For this review, take the finished solid that the model builds, in its own axes (mm). Face numbers are marked on the shaded views. A direction names the side the tool comes from. Give positions to 0.01 mm unless a question says otherwise; leave off trailing zeros. Write each loop counter-clockwise with the first axis right and the second up, starting at its lowest first coordinate (ties: lowest second). Pieces come first, ordered by that corner, then holes. Notation, with made-up numbers: (39.25, 23.25) -> (98.25, 23.25) arc R30 ccw to (98.25, 59.25) -> close; hole circle Ø4 at (-18.75, 42). An arc over 180 degrees is marked (long way). Return JSON: item names as keys, results as strings.
from build123d import *

# Parameters (mm, degrees)
F1_DEPTH = 57.15
F2_R     = 12.7
F3_DEPTH = 44.45
F4_R     = 5.08
F5_DEPTH = 25.4


with BuildPart() as f1:
    # F0 (on Front) → F1 (new body)
    with BuildSketch(Plane.XZ):
        with BuildLine():
            Line((0, 12.7), (0, 0))
            Line((0, 0), (63.5, 0))
            Line((63.5, 0), (63.5, 12.7))
            Line((63.5, 12.7), (44.45, 12.7))
            Line((44.45, 12.7), (44.45, 21.59))
            Line((44.45, 21.59), (95.25, 21.59))
            Line((95.25, 21.59), (95.25, 34.29))
            Line((95.25, 34.29), (79.375, 34.29))
            Line((79.375, 34.29), (52.843426, 73.840173))
            ThreePointArc((52.843426, 73.840173), (43.702941, 82.101765), (31.75, 85.09))
            ThreePointArc((31.75, 85.09), (19.797059, 82.101765), (10.656574, 73.840173))
            Line((10.656574, 73.840173), (-15.875, 34.29))
            Line((-15.875, 34.29), (-31.75, 34.29))
            Line((-31.75, 34.29), (-31.75, 21.59))
            Line((-31.75, 21.59), (19.05, 21.59))
            Line((19.05, 21.59), (19.05, 12.7))
            Line((19.05, 12.7), (0, 12.7))
        make_face()
        with BuildLine():
            Line((-31.75, 85.09), (-31.75, 34.29))
            Line((-31.75, 34.29), (-15.875, 34.29))
            Line((-15.875, 34.29), (10.656574, 73.840173))
            ThreePointArc((10.656574, 73.840173), (19.797059, 82.101765), (31.75, 85.09))
            Line((31.75, 85.09), (-31.75, 85.09))
        make_face()
        with BuildLine():
            Line((79.375, 34.29), (95.25, 34.29))
            Line((95.25, 34.29), (95.25, 85.09))
            Line((95.25, 85.09), (31.75, 85.09))
            ThreePointArc((31.75, 85.09), (43.702941, 82.101765), (52.843426, 73.840173))
            Line((52.843426, 73.840173), (79.375, 34.29))
        make_face()
    extrude(amount=F1_DEPTH)

    # F2 (on face) → F3 (cut)
    with BuildSketch(Plane.XZ.offset(57.15)):
        with BuildLine():
            Line((-31.75, 85.09), (-31.75, 34.29))
            Line((-31.75, 34.29), (-16.115654, 34.29))
            Line((-16.115654, 34.29), (10.664181, 74.163921))
            ThreePointArc((10.664181, 74.163921), (18.082063, 81.411466), (27.778468, 85.09))
            Line((27.778468, 85.09), (-31.75, 85.09))
        make_face()
        with BuildLine():
            Line((95.25, 85.09), (35.721532, 85.09))
            ThreePointArc((35.721532, 85.09), (45.417937, 81.411466), (52.835819, 74.163921))
            Line((52.835819, 74.163921), (79.615654, 34.29))
            Line((79.615654, 34.29), (95.25, 34.29))
            Line((95.25, 34.29), (95.25, 85.09))
        make_face()
        with BuildLine():
            ThreePointArc((35.721532, 85.09), (31.75, 85.402415), (27.778468, 85.09))
            Line((27.778468, 85.09), (35.721532, 85.09))
        make_face()
        with Locations((31.75, 60.002415)):
            Circle(F2_R)
    extrude(amount=-F3_DEPTH, mode=Mode.SUBTRACT)

    # F4 (on face) → F5 (cut)
    with BuildSketch(Plane.XY.offset(85.09)):
        with Locations((31.75, -34.925)):
            Circle(F4_R)
    extrude(amount=-F5_DEPTH, mode=Mode.SUBTRACT)


solid = f1.part
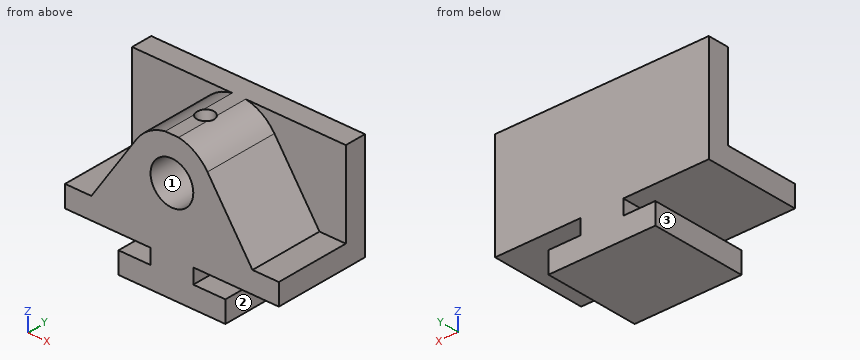
1. To check wall thickness, follow probe 1 along Z at (x, y) = (52, -8.5); probe 2 along Z at (x, y) = (31.75, -45); probe 3 along Y at (x, z) = (31.75, 75.25) (3 decimals). State the ranges of each line that lie inside material, in increasing order.
Results found:
{"probe 1": "z = 0 to 12.7, 21.59 to 85.09", "probe 2": "z = 0 to 47.3, 72.7 to 85.09", "probe 3": "y = -57.15 to -40.005, -29.845 to 0"}
2. Add section B-B, the plane y = -25. State the section outline as (x, z) points, plus the area to 3 significant figures.
Results found:
{"outline": "(-31.75, 21.59) -> (19.05, 21.59) -> (19.05, 12.7) -> (0, 12.7) -> (0, 0) -> (63.5, 0) -> (63.5, 12.7) -> (44.45, 12.7) -> (44.45, 21.59) -> (95.25, 21.59) -> (95.25, 34.29) -> (79.62, 34.29) -> (52.84, 74.16) arc R25.4 ccw to (35.72, 85.09) -> (27.78, 85.09) arc R25.4 ccw to (10.66, 74.16) -> (-16.12, 34.29) -> (-31.75, 34.29) -> close; hole circle Ø25.4 at (31.75, 60)", "area": "5,220 mm²"}
3. Add section C-C, the plane z = 11. State the section outline as (x, y) points.
Results found:
{"outline": "(0, -57.15) -> (63.5, -57.15) -> (63.5, 0) -> (0, 0) -> close"}
4. For the marked faces 1, 2 and 3, list the 3-axis set-ups (+Z, -Z, +X, -X, +Y, -Y) from which the entire face can be reached by the end or side of a thin tool; tool diameter is ignored.
Results found:
{"face 1": "-Y", "face 2": "-Z, +X, +Y, -Y", "face 3": "-Z, -X, +Y, -Y"}
5. Add section A-A, the plane x = 31.75. State the section outline as (y, z) points (3 decimals).
Results found:
{"outline": "(-57.15, 0) -> (0, 0) -> (0, 85.09) -> (-29.845, 85.09) -> (-29.845, 72.702) -> (-12.7, 72.702) -> (-12.7, 47.302) -> (-57.15, 47.302) -> close; (-57.15, 72.702) -> (-40.005, 72.702) -> (-40.005, 85.09) -> (-57.15, 85.09) -> close"}
6. For pin 1 (12 mm diameter, centred on x = 67.5, z = 58, fed in from -Y); pin 2 (4 mm diameter, centred on x = 68, z = 18, fed in from +Y); pin 3 (7 mm diameter, centred on y = -21, z = 15.5, fed in from -X); pin 4 (15 mm diameter, centred on x = 76.5, y = -34, fed in from -Z), all flat-tipped, find the tip position at first contact; note any pin that passes through.
Results found:
{"pin 1": "stops at y = -57.15", "pin 2": "passes through", "pin 3": "stops at x = 0", "pin 4": "stops at z = 21.59"}
7. Add section D-D, the plane x = 6. State the section outline as (y, z) points.
Results found:
{"outline": "(-57.15, 0) -> (0, 0) -> (0, 12.7) -> (-57.15, 12.7) -> close; (-57.15, 21.59) -> (0, 21.59) -> (0, 85.09) -> (-12.7, 85.09) -> (-12.7, 67.22) -> (-57.15, 67.22) -> close"}
